```python
from build123d import *

# Parameters (mm, degrees)
ESQUISSE1_R        = 5.1
BOSS_EXTRU_1_DEPTH = 1.6
CONG_1_R           = 3
ESQUISSE2_R        = 5.5
BOSS_EXTRU_2_DEPTH = 0.5


with BuildPart() as part:
    # Esquisse1 → Boss.-Extru.1 (new body)
    with BuildSketch(Plane.XY):
        with BuildLine():
            Line((30.049958403, 11), (20, 11))
            ThreePointArc((20, 11), (9, 0), (20, -11))
            Line((20, -11), (30.049958403, -11))
            ThreePointArc((30.049958403, -11), (0.469484965, -31.996555813), (-29.714285714, -11.876919823))
            ThreePointArc((-29.714285714, -11.876919823), (-16, 0), (-29.714285714, 11.876919823))
            ThreePointArc((-29.714285714, 11.876919823), (0.469484965, 31.996555813), (30.049958403, 11))
        make_face()
        Circle(ESQUISSE1_R, mode=Mode.SUBTRACT)
    extrude(amount=BOSS_EXTRU_1_DEPTH)

    # Congé1
    cong_1_edges = [part.edges().sort_by_distance(p)[0] for p in [
        (30.049958403, 11, 0.8),
        (30.049958403, -11, 0.8),
        (-29.714285714, -11.876919823, 0.8),
        (-29.714285714, 11.876919823, 0.8),
    ]]
    fillet(cong_1_edges, radius=CONG_1_R)

    # Esquisse2 → Boss.-Extru.2 (add)
    with BuildSketch(Plane.XY.offset(1.6)):
        with BuildLine():
            Line((20, 11.4), (25.396850198, 11.4))
            ThreePointArc((25.396850198, 11.4), (27.635538238, 12.677776168), (27.673809182, 15.255172414))
            ThreePointArc((27.673809182, 15.255172414), (0.43695488, 31.596978818), (-27.24137931, 16.014595008))
            ThreePointArc((-27.24137931, 16.014595008), (-27.375100724, 13.639159391), (-25.52, 12.149469124))
            ThreePointArc((-25.52, 12.149469124), (-15.6, 0), (-25.52, -12.149469124))
            ThreePointArc((-25.52, -12.149469124), (-27.375100724, -13.639159391), (-27.24137931, -16.014595008))
            ThreePointArc((-27.24137931, -16.014595008), (0.43695488, -31.596978818), (27.673809182, -15.255172414))
            ThreePointArc((27.673809182, -15.255172414), (27.635538238, -12.677776168), (25.396850198, -11.4))
            Line((25.396850198, -11.4), (20, -11.4))
            ThreePointArc((20, -11.4), (8.6, 0), (20, 11.4))
        make_face()
        Circle(ESQUISSE2_R, mode=Mode.SUBTRACT)
    extrude(amount=BOSS_EXTRU_2_DEPTH)


solid = part.part
```
Geometry: final body of the model. Coordinates: model frame, mm. A direction names the side the tool comes from. Give positions to 0.01 mm unless a question says otherwise; leave off trailing zeros. Order: outer loops, then holes, each group sorted by start corner. A loop starts at its lowest first (then second) coordinate and runs counter-clockwise, first axis right, second up. Notation, with made-up numbers: M 16,-17 L 75,-17 A11 cw 75,-1 Z; hole C 40.5,57 d6. An arc over 180 degrees is marked long. Answer as CSV lines item,"result". Start each with the question number.
1) Mould query, pull axis X, two halves, no side actions, for faces 5 (the cylindrical face through (2.4, -4.5, 0.8)), 6 (the cylindrical face through (9, 0, 1)), 7 (the flat face through (-21, 10, 1.6)). Classes: +X half, -X half, draft (parallel to the pull), parting line (faces both ways), or undercut.
2) Cut plane B-B (y = 0). Output: boundary loops of the cut face in (x, z).
3) Set-up query: faces 1 (the flat face through (23, -11, 1)), 2 (the cylindrical face through (-27.36, -13.61, 1.85)), 3 (the cylindrical face through (0.903, 31.587, 1.846)), 4 (the cylindrical face through (27.655, -12.71, 1.846)). Return all of +Z, -Z, +X, -X, +Y, -Y with unobstructed straight access to the full face (end or side cutting, diameter ignored); none if empty.
4) Cut plane A-A (x = 0). Output: boundary loops of the cut face in (y, z).
5) Line query: line 1 (Y direction, x = 0, z = 0.95); line 2 (Y direction, x = -3, z = 0.7); line 3 (X direction, y = 2, z = 0.75). Output: solid intervals per line, ascending. Write a range as from..to.
6) First-contact query: P1, Ø0.6, axis at x = 24, z = 2, coming from the +Y side; P2, Ø0.8, axis at x = 22.5, z = 0.5, coming from the -Y side; P3, Ø0.6, axis at x = 22.5, z = 2, coming from the -Y side. Flat tips, straight axial feed; report the tip coordinate or a pass-through.
7) Cut plane C-C (y = -22). Output: boundary loops of the cut face in (x, z).
Findings below:
1,face 5,"undercut"
1,face 6,"+X half"
1,face 7,"draft"
2,outline,"M -16,0 L -5.1,0 L -5.1,1.6 L -5.5,1.6 L -5.5,2.1 L -15.6,2.1 L -15.6,1.6 L -16,1.6 Z; M 5.1,0 L 9,0 L 9,1.6 L 8.6,1.6 L 8.6,2.1 L 5.5,2.1 L 5.5,1.6 L 5.1,1.6 Z"
3,face 1,"+Z, -Z, +X"
3,face 2,"+Z, -X"
3,face 3,"+Z, +Y"
3,face 4,"+Z, +X"
4,outline,"M -32,0 L -5.1,0 L -5.1,1.6 L -5.5,1.6 L -5.5,2.1 L -31.6,2.1 L -31.6,1.6 L -32,1.6 Z; M 5.1,0 L 32,0 L 32,1.6 L 31.6,1.6 L 31.6,2.1 L 5.5,2.1 L 5.5,1.6 L 5.1,1.6 Z"
5,line 1,"y = -32..-5.1, 5.1..32"
5,line 2,"y = -31.86..-4.12, 4.12..31.86"
5,line 3,"x = -16.17..-4.69, 4.69..9.18"
6,P1,"stops at y = 20.9"
6,P2,"stops at y = -23.14"
6,P3,"stops at y = -22.49"
7,outline,"M -23.24,0 L 23.24,0 L 23.24,1.6 L 22.68,1.6 L 22.68,2.1 L -22.68,2.1 L -22.68,1.6 L -23.24,1.6 Z"
